Read the model definition and answer for the solid it produces. Units are mm, in the model's axes. A direction names the side the tool comes from. Coordinates: 2 decimals unless noted, no trailing zeros. Order: outer loops, then holes, each group sorted by start corner. A loop starts at its lowest first (then second) coordinate and runs counter-clockwise, first axis right, second up. Notation, with made-up numbers: M 18.25,27.5 L 43.25,27.5 A9 cw 43.25,33.5 Z; hole C 16,18 d10. An arc over 180 degrees is marked long. One line per question, with ' | ' between items. Start each with the question number.
1) Find section B-B, the plane x = -15. Write down the section's boundary in (y, z).
2) The mould has two halves that part along X. Classify faces 1 (the face through (4.74, 44.4, 37.24)), 2 (the face through (-40.385, 37, 30)), 3 (the face through (-50.385, 17, 22)): +X half, -X half, draft (parallel to the pull), parting line (faces both ways), or undercut.
3) Find section A-A, the plane z = 48.5. Write down the section's boundary in (x, y), plus the area to 3 significant figures.
4) Find section C-C, the plane x = 2. Write down the section's boundary in (y, z).
5) Given P1, Ø1.5, axis at x = -1, z = 56, coming from the +Y side; P2, Ø1.5, axis at y = 18, z = 2, coming from the +X side; P3, Ø25, axis at x = -13, y = -15.5, coming from the +Z side; P4, Ø10, axis at y = 51.5, z = 42.5, coming from the -X side, each flat-ended and moving along its own axis, determine where each tip first touches the part or whether it passes through.
6) A tool of negligible diameter and unlimited length cuts with its end or side. For faces 4 (the face through (4, 18, 5)), 5 (the face through (-21, 27.639, 38)), 6 (the face through (-20.825, 17.499, 46.005)), 7 (the face through (-20, 7.639, 38)), 8 (the face through (-44, 18, 5)), from which of +Z, -Z, +X, -X, +Y, -Y can it reach the whole face along a straight path? Write none if from no direction.
7) Find section D-D, the plane y = 65. Write down the section's boundary in (x, z), plus the area to 3 significant figures.
8) Consider probe 1 along Y at (x, z) = (-15.5, 11); probe 2 along X at (y, z) = (34, 31); probe 3 along Z at (x, y) = (-35, 56). Determine where each line is inside the solid, lowest interval first.
from build123d import *

# Parameters (mm, degrees)
F0_W           = 60
F0_H           = 120
F1_DEPTH       = 20
F3_W           = 12
F3_H           = 120
F4_DEPTH       = 5
F5_R           = 8
F6_DEPTH       = 45.4
F7_W           = 60
F7_H           = 20
F8_DEPTH       = 46
F11_DEPTH      = 60
F13_DEPTH      = 212.7
F13_DEPTH_BACK = 25
F15_DEPTH      = 46


with BuildPart() as f1:
    # F0 (on Top) → F1 (new body)
    with BuildSketch(Plane.XY):
        with Locations((-20.3850728273, 17.6392173767)):
            Rectangle(F0_W, F0_H)
    extrude(amount=F1_DEPTH)

    # F3 (on face) → F4 (cut)
    with BuildSketch(Plane.XY):
        with Locations((-44.3850728273, 17.6392173767)):
            Rectangle(F3_W, F3_H)
        with Locations((3.6149271727, 17.6392173767)):
            Rectangle(F3_W, F3_H)
    extrude(amount=F4_DEPTH, mode=Mode.SUBTRACT)

    # F5 (on face) → F6 (cut)
    with BuildSketch(Plane.XY.offset(20)):
        with BuildLine():
            ThreePointArc((-20.3850728273, -9.3607826233), (-28.3850728273, -17.3607826233), (-20.3850728273, -25.3607826233))
            Line((-20.3850728273, -25.3607826233), (-20.3850728273, -17.3607826233))
            Line((-20.3850728273, -17.3607826233), (-20.3850728273, -9.3607826233))
        make_face()
        with BuildLine():
            Line((-20.3850728273, -17.3607826233), (-20.3850728273, -25.3607826233))
            ThreePointArc((-20.3850728273, -25.3607826233), (-14.7282185778, -23.0176368728), (-12.3850728273, -17.3607826233))
            Line((-12.3850728273, -17.3607826233), (-20.3850728273, -17.3607826233))
        make_face()
        with BuildLine():
            Line((-20.3850728273, -9.3607826233), (-20.3850728273, -17.3607826233))
            Line((-20.3850728273, -17.3607826233), (-12.3850728273, -17.3607826233))
            ThreePointArc((-12.3850728273, -17.3607826233), (-14.7282185778, -11.7039283738), (-20.3850728273, -9.3607826233))
        make_face()
        with Locations((-20.3850728273, 52.6392173767)):
            Circle(F5_R)
    extrude(amount=-F6_DEPTH, mode=Mode.SUBTRACT)

    # F7 (on face) → F8 (join)
    with BuildSketch(Plane.XY.offset(20)):
        with Locations((-20.3850728273, 17.6392173767)):
            Rectangle(F7_W, F7_H)
    extrude(amount=F8_DEPTH)

    # F10 (on face) → F11 (join)
    with BuildSketch(Plane(origin=(-50.3850728273, 0, 0), x_dir=(0, -1, 0), z_dir=(-1, 0, 0))):
        Polygon((-7.6392173767, 20), (26.3607826233, 20), (-7.6392173767, 54), align=None)
        Polygon((-27.6392173767, 54), (-61.6392173767, 20), (-27.6392173767, 20), align=None)
    extrude(amount=-F11_DEPTH)

    # F12 (on face) → F13 (cut, two sides)
    with BuildSketch(Plane.XZ.offset(-7.6392173767)) as f13_sk:
        with BuildLine():
            ThreePointArc((-40.3850728273, 66), (-20.3850728273, 46), (-0.3850728273, 66))
            Line((-0.3850728273, 66), (-40.3850728273, 66))
        make_face()
        with BuildLine():
            Line((-40.3850728273, 66), (-0.3850728273, 66))
            ThreePointArc((-0.3850728273, 66), (-20.3850728273, 86), (-40.3850728273, 66))
        make_face()
    extrude(amount=-F13_DEPTH, mode=Mode.SUBTRACT)
    extrude(f13_sk.sketch, amount=F13_DEPTH_BACK, mode=Mode.SUBTRACT)

    # F14 (on face) → F15 (cut, through all)
    with BuildSketch(Plane.XY.offset(66)):
        Polygon((-40.3850728273, 61.7061406374), (-40.3850728273, 27.6392173767), (-0.3850728273, 27.6392173767), (0, 27.6392173767), (0, 61.7061406374), align=None)
        Polygon((-0.3850728273, 7.6392173767), (-40.3850728273, 7.6392173767), (-40.3850728273, -26.4050289989), (0, -26.4050289989), (0, 7.6392173767), align=None)
    extrude(amount=-F15_DEPTH, mode=Mode.SUBTRACT)


solid = f1.part
Report:
1) outline: M -42.36,0 L -23.28,0 L -23.28,20 L -42.36,20 Z; M -11.44,0 L 46.72,0 L 46.72,20 L 27.64,20 L 27.64,46.74 L 7.64,46.74 L 7.64,20 L -11.44,20 Z; M 58.56,0 L 77.64,0 L 77.64,20 L 58.56,20 Z
2) face 1: draft | face 2: undercut | face 3: -X half
3) outline: M -50.39,2.14 L -40.39,2.14 L -40.39,7.64 L -30.07,7.64 L -30.07,27.64 L -40.39,27.64 L -40.39,33.14 L -50.39,33.14 Z; M -10.7,7.64 L 0,7.64 L 0,2.14 L 9.61,2.14 L 9.61,33.14 L 0,33.14 L 0,27.64 L -10.7,27.64 Z | area: 1,030 mm^2
4) outline: M -42.36,5 L 77.64,5 L 77.64,20 L 61.64,20 L 27.64,54 L 27.64,66 L 7.64,66 L 7.64,54 L -26.36,20 L -42.36,20 Z
5) P1: stops at y = 27.64 | P2: stops at x = -2.39 | P3: stops at z = 20 | P4: passes through
6) face 4: -Z, +X, +Y, -Y | face 5: +Z, +Y | face 6: +Z, +Y, -Y | face 7: +Z, -Y | face 8: -Z, -X, +Y, -Y
7) outline: M -50.39,5 L -38.39,5 L -38.39,0 L -2.39,0 L -2.39,5 L 9.61,5 L 9.61,20 L -50.39,20 Z | area: 1,080 mm^2
8) probe 1: y = -42.36 to -23.7, -11.03 to 46.3, 58.97 to 77.64 | probe 2: x = -50.39 to -40.39, 0 to 9.61 | probe 3: z = 0 to 20
